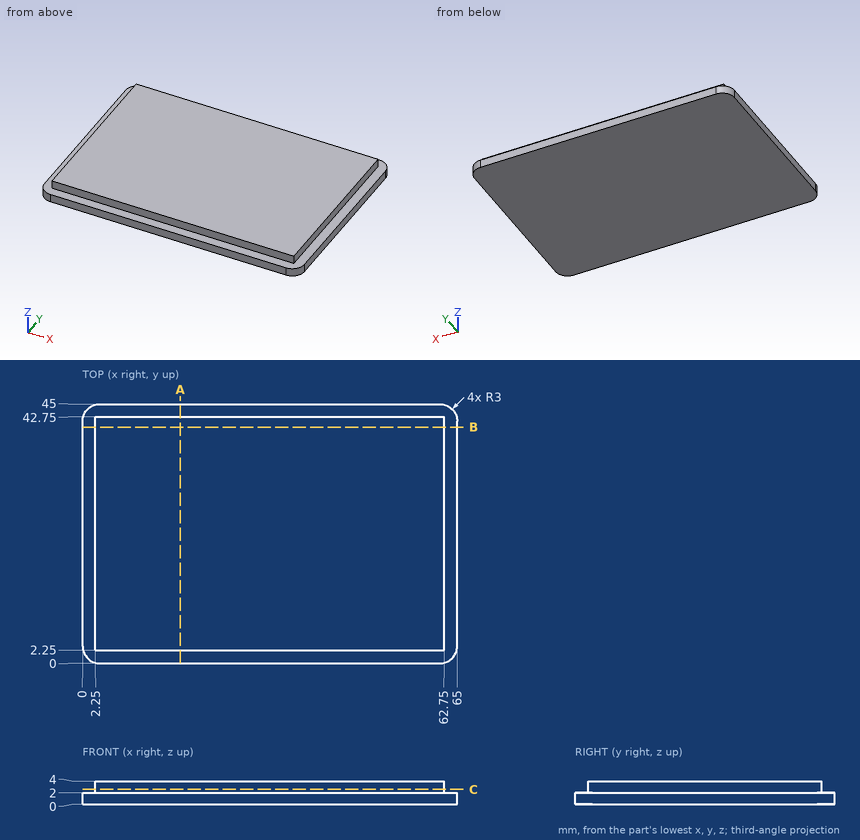
Check sheet for the drawn part. Datum: minimum x, y, z corner. Units: mm. Round coordinates to 2 decimals unless told otherwise and drop trailing zeros. Loops run counter-clockwise (first coordinate to the right, second up) from the corner with the lowest first, then second, coordinate; pieces in that order, holes last. Notation, with made-up numbers: (34.5, 15) - (73.5, 15) arc R29 ccw to (73.5, 50) - close; hole circle Ø6 at (-9, 52). An arc over 180 degrees is marked (long way). Write each question's results on one line, items separated by ' | '. Start each with the question number.
Q1. Cross-section at C-C on z = 2.6. Enter the section's corners in (x, y), and give its area (3 significant figures).
Q2. Thickness scan on line 1 (Y direction, x = 10, z = 3.7); line 2 (X direction, y = 16.5, z = 2.4). Record the ranges inside material, lowest first. Write a range as [from, to].
Q3. Gauge pin test, flat ends, axial feed: P1, Ø1.6, axis at y = 19.5, z = 3, coming from the +X side; P2, Ø2, axis at x = 38.5, z = 3.5, coming from the +Y side. Record the tip position at first contact, or that the pin passes through.
Q4. Cross-section at B-B on y = 41. Enter the section's corners in (x, z).
Q5. Cross-section at A-A on x = 17. Enter the section's corners in (y, z), and give its area (3 significant figures).
Answers below:
1) outline: (2.25, 2.25) - (62.75, 2.25) - (62.75, 42.75) - (2.25, 42.75) - close | area: 2,450 mm²
2) line 1: y = [2.25, 42.75] | line 2: x = [2.25, 62.75]
3) P1: stops at x = 62.75 | P2: stops at y = 42.75
4) outline: (0, 0) - (65, 0) - (65, 2) - (62.75, 2) - (62.75, 4) - (2.25, 4) - (2.25, 2) - (0, 2) - close
5) outline: (0, 0) - (45, 0) - (45, 2) - (42.75, 2) - (42.75, 4) - (2.25, 4) - (2.25, 2) - (0, 2) - close | area: 171 mm²
